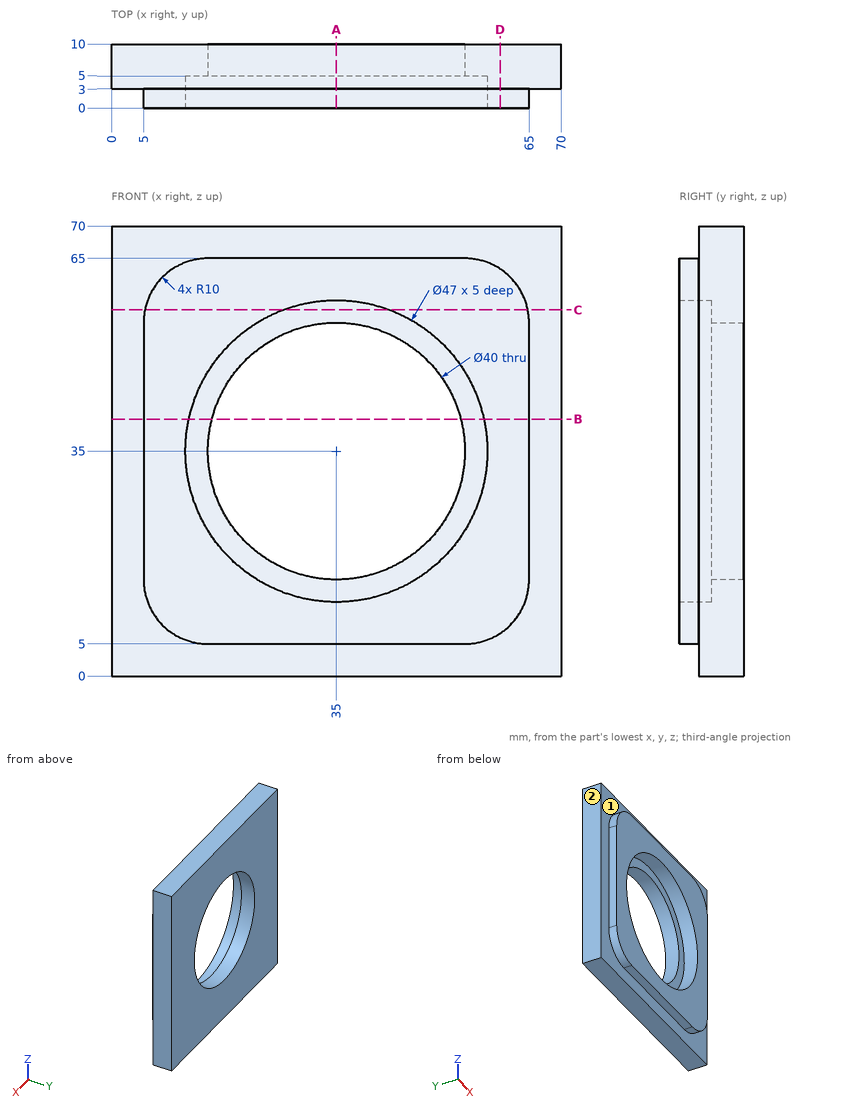
Job drawing, mm, ordinate dimensions from the low corner. One solid piece. A direction names the side the tool comes from. Round coordinates to 2 decimals unless told otherwise and drop trailing zeros. Write each loop counter-clockwise with the first axis right and the second up, starting at its lowest first coordinate (ties: lowest second). Pieces come first, ordered by that corner, then holes.
1) Band-saw the part on B-B, the plane z = 40. List the corners of the cut face in (x, y).
2) Band-saw the part on C-C, the plane z = 57. List the corners of the cut face in (x, y).
3) Band-saw the part on D-D, the plane x = 60.5. List the corners of the cut face in (y, z), and give its area (3 significant figures).
4) Drill centre lines: probe 1 along X at (y, z) = (3.75, 35); probe 2 along X at (y, z) = (8.55, 35); probe 3 along Z at (x, y) = (53.5, 1.75). Where is each one in solid material? Low to high.
5) Pin check, flat tips, straight feed: pin 1 (1.5 mm diameter, centred on x = 34, y = 1, fed in from +Z); pin 2 (1.5 mm diameter, centred on x = 36.5, y = 2, fed in from -Z); pin 3 (23.5 mm diameter, centred on x = 28.5, z = 25.5, fed in from -Y). Stop position of each tip, or through.
6) 3-axis set-ups, long thin cutter, end or side, ignore diameter. For the marked faces 1 and 2: which of +Z, -Z, +X, -X, +Y, -Y reach the whole face in a straight line?
7) Band-saw the part on A-A, the plane x = 35. List the corners of the cut face in (y, z), and give its area (3 significant figures).
Ans:
1. outline: (0, 3) - (5, 3) - (5, 0) - (12.04, 0) - (12.04, 5) - (15.64, 5) - (15.64, 10) - (0, 10) - close; (54.36, 5) - (57.96, 5) - (57.96, 0) - (65, 0) - (65, 3) - (70, 3) - (70, 10) - (54.36, 10) - close
2. outline: (0, 3) - (5.2, 3) - (5.2, 0) - (26.74, 0) - (26.74, 5) - (43.26, 5) - (43.26, 0) - (64.8, 0) - (64.8, 3) - (70, 3) - (70, 10) - (0, 10) - close
3. outline: (0, 6.65) - (3, 6.65) - (3, 0) - (10, 0) - (10, 70) - (3, 70) - (3, 63.35) - (0, 63.35) - close
3. area: 660 mm2
4. probe 1: x = 0 to 11.5, 58.5 to 70
4. probe 2: x = 0 to 15, 55 to 70
4. probe 3: z = 5 to 20.51, 49.49 to 65
5. pin 1: stops at z = 65
5. pin 2: stops at z = 5
5. pin 3: stops at y = 5
6. face 1: -Y
6. face 2: +Z, -Z, -X, +Y, -Y
7. outline: (0, 5) - (3, 5) - (3, 0) - (10, 0) - (10, 15) - (5, 15) - (5, 11.5) - (0, 11.5) - close; (0, 58.5) - (5, 58.5) - (5, 55) - (10, 55) - (10, 70) - (3, 70) - (3, 65) - (0, 65) - close
7. area: 235 mm2
